Geometry: final body of the model. Coordinates: model frame, mm. A direction names the side the tool comes from. Give positions to 0.01 mm unless a question says otherwise; leave off trailing zeros. Loops run counter-clockwise (first coordinate to the right, second up) from the corner with the lowest first, then second, coordinate; pieces in that order, holes last.
from build123d import *

# Parameters (mm, degrees)
SKETCH_1_R          = 39.5
EXTRUDE_1_DEPTH     = 14
SKETCH_2_R          = 2.25
SKETCH_2_R_2        = 2
CUT_EXTRUDE_1_DEPTH = 16
CUT_EXTRUDE_2_DEPTH = 4
CUT_EXTRUDE_3_DEPTH = 4
SKETCH_8_R          = 24.05
CUT_EXTRUDE_4_DEPTH = 9
SKETCH_9_R          = 2.5
CUT_EXTRUDE_5_DEPTH = 15
SKETCH_10_R         = 19.125
EXTRUDE_2_DEPTH     = 5
SKETCH_11_R         = 13
CUT_EXTRUDE_6_DEPTH = 104
CUT_EXTRUDE_7_DEPTH = 5
CHAMFER_2_SIZE      = 0.6
CHAMFER_3_SIZE      = 0.6
CHAMFER_4_SIZE      = 0.6
CHAMFER_5_SIZE      = 0.6
CHAMFER_6_SIZE      = 0.6
CHAMFER_7_SIZE      = 0.6
CHAMFER_9_SIZE      = 0.6
CHAMFER_10_SIZE     = 0.6
CHAMFER_11_SIZE     = 0.6
CHAMFER_12_SIZE     = 0.6


with BuildPart() as part:
    # 草图1 → 凸台-拉伸1 (new body)
    with BuildSketch(Plane(origin=(0, 0, 0), x_dir=(0, 0, -1), z_dir=(1, 0, 0))):
        Circle(SKETCH_1_R)
    extrude(amount=EXTRUDE_1_DEPTH)

    # 草图2 → 切除-拉伸1 (cut)
    with BuildSketch(Plane.ZY):
        with Locations((-35.5, 0)):
            Circle(SKETCH_2_R)
        with Locations((-30.743901834, 17.75)):
            Circle(SKETCH_2_R_2)
        with Locations((-17.75, 30.743901834)):
            Circle(SKETCH_2_R)
        with Locations((0, 35.5)):
            Circle(SKETCH_2_R_2)
        with Locations((17.75, 30.743901834)):
            Circle(SKETCH_2_R)
        with Locations((30.743901834, 17.75)):
            Circle(SKETCH_2_R_2)
        with Locations((35.5, 0)):
            Circle(SKETCH_2_R)
        with Locations((30.743901834, -17.75)):
            Circle(SKETCH_2_R_2)
        with Locations((17.75, -30.743901834)):
            Circle(SKETCH_2_R)
        with Locations((0, -35.5)):
            Circle(SKETCH_2_R_2)
        with Locations((-17.75, -30.743901834)):
            Circle(SKETCH_2_R)
        with Locations((-30.743901834, -17.75)):
            Circle(SKETCH_2_R_2)
    extrude(amount=-CUT_EXTRUDE_1_DEPTH, mode=Mode.SUBTRACT)

    # 草图4 → 切除-拉伸2 (cut)
    with BuildSketch(Plane(origin=(14, 0, 0), x_dir=(0, 0, -1), z_dir=(1, 0, 0))):
        with BuildLine():
            Line((-35.5, 4), (-44.201093629, 4))
            Line((-44.201093629, 4), (-44.201093629, -4))
            Line((-44.201093629, -4), (-35.5, -4))
            ThreePointArc((-35.5, -4), (-31.5, 0), (-35.5, 4))
        make_face()
    extrude(amount=-CUT_EXTRUDE_2_DEPTH, mode=Mode.SUBTRACT)

    # 草图7 → 切除-拉伸3 (cut)
    with BuildSketch(Plane(origin=(14, 0, 0), x_dir=(0, 0, -1), z_dir=(1, 0, 0))):
        with BuildLine():
            Line((-21.214101615, -28.743901834), (-24.616312288, -34.636703577))
            Line((-24.616312288, -34.636703577), (-17.688109058, -38.636703577))
            Line((-17.688109058, -38.636703577), (-14.285898385, -32.743901834))
            ThreePointArc((-14.285898385, -32.743901834), (-15.75, -27.279800219), (-21.214101615, -28.743901834))
        make_face()
        with BuildLine():
            Line((14.285898385, -32.743901834), (17.598294891, -38.481140877))
            Line((17.598294891, -38.481140877), (24.526498121, -34.481140877))
            Line((24.526498121, -34.481140877), (21.214101615, -28.743901834))
            ThreePointArc((21.214101615, -28.743901834), (15.75, -27.279800219), (14.285898385, -32.743901834))
        make_face()
        with BuildLine():
            Line((35.5, -4), (41.305115607, -4))
            Line((41.305115607, -4), (41.305115607, 4))
            Line((41.305115607, 4), (35.5, 4))
            ThreePointArc((35.5, 4), (31.5, 0), (35.5, -4))
        make_face()
        with BuildLine():
            Line((21.214101615, 28.743901834), (23.957184481, 33.495060727))
            Line((23.957184481, 33.495060727), (17.02898125, 37.495060727))
            Line((17.02898125, 37.495060727), (14.285898385, 32.743901834))
            ThreePointArc((14.285898385, 32.743901834), (15.75, 27.279800219), (21.214101615, 28.743901834))
        make_face()
        with BuildLine():
            Line((-14.285898385, 32.743901834), (-17.02898125, 37.495060727))
            Line((-17.02898125, 37.495060727), (-23.957184481, 33.495060727))
            Line((-23.957184481, 33.495060727), (-21.214101615, 28.743901834))
            ThreePointArc((-21.214101615, 28.743901834), (-15.75, 27.279800219), (-14.285898385, 32.743901834))
        make_face()
    extrude(amount=-CUT_EXTRUDE_3_DEPTH, mode=Mode.SUBTRACT)

    # 草图8 → 切除-拉伸4 (cut)
    with BuildSketch(Plane.ZY):
        Circle(SKETCH_8_R)
    extrude(amount=-CUT_EXTRUDE_4_DEPTH, mode=Mode.SUBTRACT)

    # 草图9 → 切除-拉伸5 (cut)
    with BuildSketch(Plane(origin=(14, 0, 0), x_dir=(0, 0, -1), z_dir=(1, 0, 0))):
        with Locations((23.55, -23.55)):
            Circle(SKETCH_9_R)
        with Locations((-23.55, -23.55)):
            Circle(SKETCH_9_R)
        with Locations((-23.55, 23.55)):
            Circle(SKETCH_9_R)
        with Locations((23.55, 23.55)):
            Circle(SKETCH_9_R)
    extrude(amount=-CUT_EXTRUDE_5_DEPTH, mode=Mode.SUBTRACT)

    # 草图10 → 凸台-拉伸2 (add)
    with BuildSketch(Plane(origin=(14, 0, 0), x_dir=(0, 0, -1), z_dir=(1, 0, 0))):
        Circle(SKETCH_10_R)
    extrude(amount=EXTRUDE_2_DEPTH)

    # 草图11 → 切除-拉伸6 (cut)
    with BuildSketch(Plane(origin=(19, 0, 0), x_dir=(0, 0, -1), z_dir=(1, 0, 0))):
        Circle(SKETCH_11_R)
    extrude(amount=-CUT_EXTRUDE_6_DEPTH, mode=Mode.SUBTRACT)

    # 草图12 → 切除-拉伸7 (cut)
    with BuildSketch(Plane.ZY):
        with BuildLine():
            Line((20.014466094, -27.085533906), (26.013985292, -33.085053103))
            Line((26.013985292, -33.085053103), (33.085053103, -26.013985292))
            Line((33.085053103, -26.013985292), (27.085533906, -20.014466094))
            ThreePointArc((27.085533906, -20.014466094), (20.014466094, -20.014466094), (20.014466094, -27.085533906))
        make_face()
        with BuildLine():
            Line((27.085533906, 20.014466094), (32.930330591, 25.859262779))
            Line((32.930330591, 25.859262779), (25.859262779, 32.930330591))
            Line((25.859262779, 32.930330591), (20.014466094, 27.085533906))
            ThreePointArc((20.014466094, 27.085533906), (20.014466094, 20.014466094), (27.085533906, 20.014466094))
        make_face()
        with BuildLine():
            Line((-20.014466094, 27.085533906), (-27.290112032, 34.361179844))
            Line((-27.290112032, 34.361179844), (-34.361179844, 27.290112032))
            Line((-34.361179844, 27.290112032), (-27.085533906, 20.014466094))
            ThreePointArc((-27.085533906, 20.014466094), (-20.014466094, 20.014466094), (-20.014466094, 27.085533906))
        make_face()
        with BuildLine():
            Line((-27.085533906, -20.014466094), (-33.971209247, -26.900141436))
            Line((-33.971209247, -26.900141436), (-26.900141436, -33.971209247))
            Line((-26.900141436, -33.971209247), (-20.014466094, -27.085533906))
            ThreePointArc((-20.014466094, -27.085533906), (-20.014466094, -20.014466094), (-27.085533906, -20.014466094))
        make_face()
    extrude(amount=-CUT_EXTRUDE_7_DEPTH, mode=Mode.SUBTRACT)

    # 倒角2
    chamfer_2_edges = [part.edges().sort_by_distance(p)[0] for p in [
        (0, 12.771209477, -37.378419021),
    ]]
    chamfer(chamfer_2_edges, length=CHAMFER_2_SIZE)

    # 倒角3
    chamfer_3_edges = [part.edges().sort_by_distance(p)[0] for p in [
        (0, -39.5, 0),
    ]]
    chamfer(chamfer_3_edges, length=CHAMFER_3_SIZE)

    # 倒角4
    chamfer_4_edges = [part.edges().sort_by_distance(p)[0] for p in [
        (0, 0, 39.5),
    ]]
    chamfer(chamfer_4_edges, length=CHAMFER_4_SIZE)

    # 倒角5
    chamfer_5_edges = [part.edges().sort_by_distance(p)[0] for p in [
        (0, 39.5, 0),
    ]]
    chamfer(chamfer_5_edges, length=CHAMFER_5_SIZE)

    # 倒角6
    chamfer_6_edges = [part.edges().sort_by_distance(p)[0] for p in [
        (14, 19.75, -34.208003449),
    ]]
    chamfer(chamfer_6_edges, length=CHAMFER_6_SIZE)

    # 倒角7
    chamfer_7_edges = [part.edges().sort_by_distance(p)[0] for p in [
        (14, 39.5, 0),
    ]]
    chamfer(chamfer_7_edges, length=CHAMFER_7_SIZE)

    # 倒角9
    chamfer_9_edges = [part.edges().sort_by_distance(p)[0] for p in [
        (14, -19.75, -34.208003449),
    ]]
    chamfer(chamfer_9_edges, length=CHAMFER_9_SIZE)

    # 倒角10
    chamfer_10_edges = [part.edges().sort_by_distance(p)[0] for p in [
        (14, -39.5, 0),
    ]]
    chamfer(chamfer_10_edges, length=CHAMFER_10_SIZE)

    # 倒角11
    chamfer_11_edges = [part.edges().sort_by_distance(p)[0] for p in [
        (14, -19.75, 34.208003449),
    ]]
    chamfer(chamfer_11_edges, length=CHAMFER_11_SIZE)

    # 倒角12
    chamfer_12_edges = [part.edges().sort_by_distance(p)[0] for p in [
        (14, 19.75, 34.208003449),
    ]]
    chamfer(chamfer_12_edges, length=CHAMFER_12_SIZE)


solid = part.part
Item 1: Section query C-C on x = 16.5. Return loops of the section in (y, z) (3 decimals).
Values follow:
outline: circle Ø38.25 at (0, 0); hole circle Ø26 at (0, 0)
Item 2: Section query A-A on z = 0. Return loops of the section in (x, y) (3 decimals).
Values follow:
outline: (0, -38.9) - (0.6, -39.5) - (13.4, -39.5) - (14, -38.9) - (14, -37.5) - (0, -37.5) - close; (0, -33.5) - (14, -33.5) - (14, -19.125) - (19, -19.125) - (19, -13) - (9, -13) - (9, -24.05) - (0, -24.05) - close; (0, 24.05) - (9, 24.05) - (9, 13) - (19, 13) - (19, 19.125) - (14, 19.125) - (14, 33.5) - (0, 33.5) - close; (0, 37.5) - (14, 37.5) - (14, 38.9) - (13.4, 39.5) - (0.6, 39.5) - (0, 38.9) - close
Item 3: Set-up query: faces 5 (the face through (12, 4, 37)), 6 (the face through (10, 32.5, -19.4)), 7 (the face through (12.028, 30.411, 22.177)), 8 (the face through (10, -2, -37)). Return all of +Z, -Z, +X, -X, +Y, -Y with unobstructed straight access to the full face (end or side cutting, diameter ignored); none if empty.
Values follow:
face 5: +Z, +X
face 6: +X
face 7: +X, +Y
face 8: -Z, +X
Item 4: Pin query (flat end, axial travel): pin 1 (2.5 mm diameter, centred on y = 0, z = -34, fed in from +X); pin 2 (10 mm diameter, centred on x = 3.5, y = 6, fed in from +Z); pin 3 (4 mm diameter, centred on x = 11, z = -37.5, fed in from -Y). Return the tip coordinate at first contact, or that it passes through.
Values follow:
pin 1: stops at x = 10
pin 2: stops at z = 39.49
pin 3: stops at y = -17.32
Item 5: Section query B-B on x = 6.5. Give the number of separate pieces and of enclosed holes in the cut face, plus the area to 3 significant figures.
Values follow:
separate pieces: 1
enclosed holes: 17
area: 2,840 mm2
Item 6: Ray query, probe 1 along Y at (x, z) = (6.25, 0); probe 2 along Y at (x, z) = (12, 23.55); probe 3 along X at (y, z) = (27.5, 14.5). Return the intervals inside material, ascending.
Values follow:
probe 1: y = -39.5 to -37.5, -33.5 to -24.05, 24.05 to 33.5, 37.5 to 39.5
probe 2: y = -31.71 to -26.05, -21.05 to 21.05, 26.05 to 31.71
probe 3: x = 0 to 14
Item 7: Draft query along Y for faces 1 (the face through (14, 18, -8)), 2 (the face through (13.84, 19.73, 33.71)), 3 (the face through (6.9, 19.1, 29.27)), 4 (the face through (13.84, -19.73, -33.71)). Return one class per face: +Y half, -Y half, draft (parallel to the pull), parting line (faces both ways), or undercut.
Values follow:
face 1: draft
face 2: +Y half
face 3: undercut
face 4: -Y half
